Could you check a few things on this drawing? It's one solid part, dimensions in mm from its lowest x, y, z. Coordinates: 2 decimals unless noted, no trailing zeros. Order: outer loops, then holes, each group sorted by start corner. A loop starts at its lowest first (then second) coordinate and runs counter-clockwise, first axis right, second up. Notation, with made-up numbers: (17.5, -37) - (44.5, -37) arc R24 ccw to (44.5, -18) - close; hole circle Ø2 at (8, 19.25). An arc over 180 degrees is marked (long way). Return JSON: item names as keys, results as strings. Group by question number.
1) Imagine slicing it at A-A (z = 20). Write out the boundary of the cut face in (x, y), and give its area (3 significant figures).
2) Imagine slicing it at B-B (x = 45). Write out the boundary of the cut face in (y, z).
3) If I drill on line 1 along X through (y, z) = (5.75, 20); line 2 along Z through (x, y) = (15, 4.5); line 3 along X through (y, z) = (6.5, 20.5), over which ranges is the centre line in solid material (lowest first)?
4) For pin 1 Ø4.5 at (x, z) = (15, 20) entering from -Y, with a flat end and sliding along its axis, tell me the tip position at first contact or that it passes through.
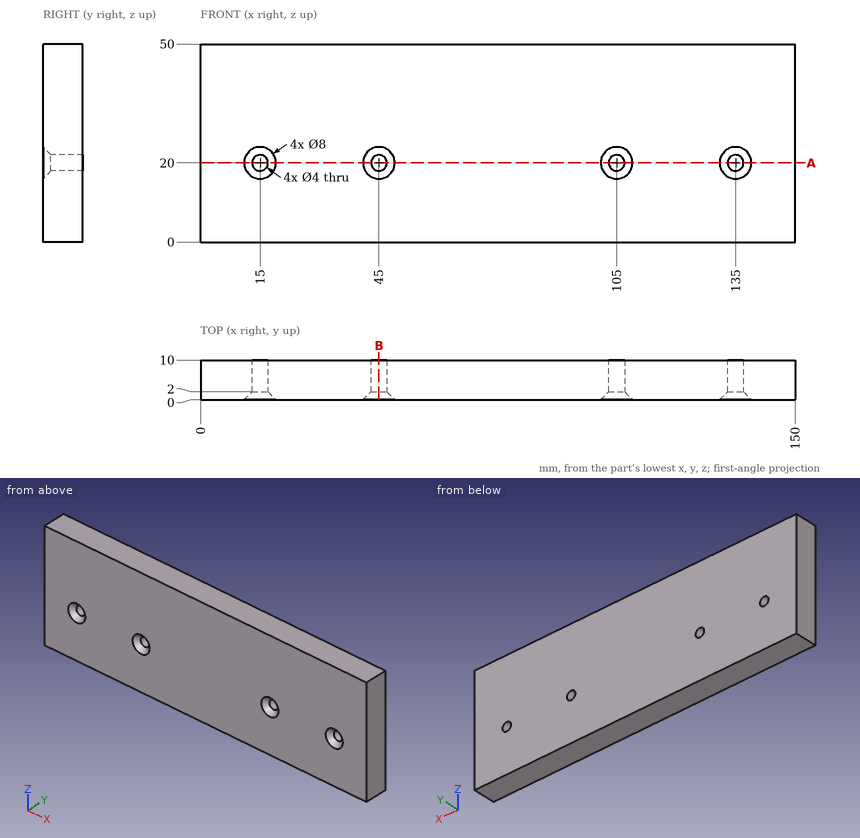
Calculated:
{
 "1": {"outline": "(0, 0) - (11, 0) - (13, 2) - (13, 10) - (0, 10) - close; (17, 2) - (19, 0) - (41, 0) - (43, 2) - (43, 10) - (17, 10) - close; (47, 2) - (49, 0) - (101, 0) - (103, 2) - (103, 10) - (47, 10) - close; (107, 2) - (109, 0) - (131, 0) - (133, 2) - (133, 10) - (107, 10) - close; (137, 2) - (139, 0) - (150, 0) - (150, 10) - (137, 10) - close", "area": "1,320 mm2"},
 "2": {"outline": "(0, 0) - (10, 0) - (10, 18) - (2, 18) - (0, 16) - close; (0, 24) - (2, 22) - (10, 22) - (10, 50) - (0, 50) - close"},
 "3": {"line 1": "0 to 13, 17 to 43, 47 to 103, 107 to 133, 137 to 150", "line 2": "0 to 18, 22 to 50", "line 3": "0 to 13.06, 16.94 to 43.06, 46.94 to 103.06, 106.94 to 133.06, 136.94 to 150"},
 "4": {"pin 1": "y = 1.75"}
}
